```python
from build123d import *

# Parameters (mm, degrees)
F0_W     = 11.43
F0_H     = 11.43
F0_W_2   = 3.81
F0_H_2   = 3.81
F1_DEPTH = 152.4
F2_W     = 3.81
F2_H     = 144.78
F3_DEPTH = 25.4
F4_W     = 3.81
F4_H     = 144.78
F5_DEPTH = 25.4


with BuildPart() as f1:
    # F0 (on Top) → F1 (new body)
    with BuildSketch(Plane.XY):
        with Locations((-54.323498, -23.599323)):
            Rectangle(F0_W, F0_H)
        with Locations((-54.323498, -23.599323)):
            Rectangle(F0_W_2, F0_H_2, mode=Mode.SUBTRACT)
    extrude(amount=F1_DEPTH)

    # F2 (on face) → F3 (cut)
    with BuildSketch(Plane(origin=(-60.038498, 0, 0), x_dir=(0, -1, 0), z_dir=(-1, 0, 0))):
        with Locations((23.599323, 76.2)):
            Rectangle(F2_W, F2_H)
    extrude(amount=-F3_DEPTH, mode=Mode.SUBTRACT)

    # F4 (on face) → F5 (cut)
    with BuildSketch(Plane(origin=(0, -17.884323, 0), x_dir=(-1, 0, 0), z_dir=(0, 1, 0))):
        with Locations((54.323498, 76.2)):
            Rectangle(F4_W, F4_H)
    extrude(amount=-F5_DEPTH, mode=Mode.SUBTRACT)


solid = f1.part
```
Verification items for the finished model (mm, model axes). A direction names the side the tool comes from. Coordinates: 2 decimals unless noted, no trailing zeros. Loops run counter-clockwise (first coordinate to the right, second up) from the corner with the lowest first, then second, coordinate; pieces in that order, holes last. Notation, with made-up numbers: (-25, -24) - (-5, -24) arc R8 cw to (-5, -19) - close; hole circle Ø7 at (23, 72). An arc over 180 degrees is marked (long way). Return JSON: item names as keys, results as strings.
1. Section check A-A, the plane z = 41.5. Record the boundary of the cut face in (x, y), then the cut area to 3 significant figures.
Established:
{"outline": "(-60.04, -29.31) - (-56.23, -29.31) - (-56.23, -25.5) - (-60.04, -25.5) - close; (-60.04, -21.69) - (-56.23, -21.69) - (-56.23, -17.88) - (-60.04, -17.88) - close; (-52.42, -29.31) - (-48.61, -29.31) - (-48.61, -25.5) - (-52.42, -25.5) - close; (-52.42, -21.69) - (-48.61, -21.69) - (-48.61, -17.88) - (-52.42, -17.88) - close", "area": "58.1 mm2"}
2. Thickness scan on L1, parallel to X at y = -19.5, z = 52.5; L2, parallel to Z at x = -57.75, y = -22.5; L3, parallel to Y at x = -51, z = 120. Record the ranges inside material, lowest first.
Established:
{"L1": "x = -60.04 to -56.23, -52.42 to -48.61", "L2": "z = 0 to 3.81, 148.59 to 152.4", "L3": "y = -29.31 to -25.5, -21.69 to -17.88"}
3. Section check B-B, the plane x = -54. Record the boundary of the cut face in (y, z), then the cut area to 3 significant figures.
Established:
{"outline": "(-29.31, 0) - (-25.5, 0) - (-25.5, 3.81) - (-29.31, 3.81) - close; (-29.31, 148.59) - (-25.5, 148.59) - (-25.5, 152.4) - (-29.31, 152.4) - close; (-21.69, 0) - (-17.88, 0) - (-17.88, 3.81) - (-21.69, 3.81) - close; (-21.69, 148.59) - (-17.88, 148.59) - (-17.88, 152.4) - (-21.69, 152.4) - close", "area": "58.1 mm2"}
4. Tool access check on faces 5 (the flat face through (-51, -24, 3.81)), 6 (the flat face through (-54, -27, 148.59)), 7 (the flat face through (-54, -25.504, 2)). Record the directions out of +Z, -Z, +X, -X, +Y, -Y that give a thin tool (end or side, any length) a straight path to the whole face; none if there is none.
Established:
{"face 5": "+X, -X", "face 6": "+Y, -Y", "face 7": "+Z, -Z"}
5. Mould release check, pull along Z, two halves, no side actions. Record for faces 1 (the flat face through (-56.228, -24, 2)), 2 (the flat face through (-52, -24, 152.4)), 3 (the flat face through (-51, -25.504, 75)), 4 (the flat face through (-52.418, -20, 75)): +Z half, -Z half, draft (parallel to the pull), parting line (faces both ways), or undercut.
Established:
{"face 1": "draft", "face 2": "+Z half", "face 3": "undercut", "face 4": "undercut"}
